Part print with two shaded views. Sizes in mm from the minimum x, y, z corner. A direction names the side the tool comes from. Round coordinates to 2 decimals unless told otherwise and drop trailing zeros. Loops run counter-clockwise (first coordinate to the right, second up) from the corner with the lowest first, then second, coordinate; pieces in that order, holes last. Notation, with made-up numbers: M -40,73.25 L -28,73.25 A29 ccw -28,108.25 Z; hole C 73,49 d11. An arc over 180 degrees is marked long. Use a Markdown table: item, result. Add a question column.
Item 1: Saw through at C-C on z = 4.25. Write the cut outline in (x, y), then the cut area to 3 significant figures.
Item 2: Tool access for the marked faces 1 and 2: list every direction of +Z, -Z, +X, -X, +Y, -Y with a clear straight run to the whole face (end or side of a thin tool).
Item 3: Pin check, flat tip, straight feed: P1, Ø3, axis at x = 4.5, z = 5, coming from the +Y side. Stop position of the tip, or through.
Item 4: Saw through at A-A on y = 2.6. Write the cut outline in (x, z).
Item 5: Wall check: L1, parallel to Y at x = 2.5, z = 6.5; L2, parallel to Z at x = 4.95, y = 1.6; L3, parallel to Y at x = 4.9, z = 2.75. Give the ranges that are in metal, low to high. Write a range as from..to.
Item 6: Saw through at D-D on z = 5.5. Write the cut outline in (x, y).
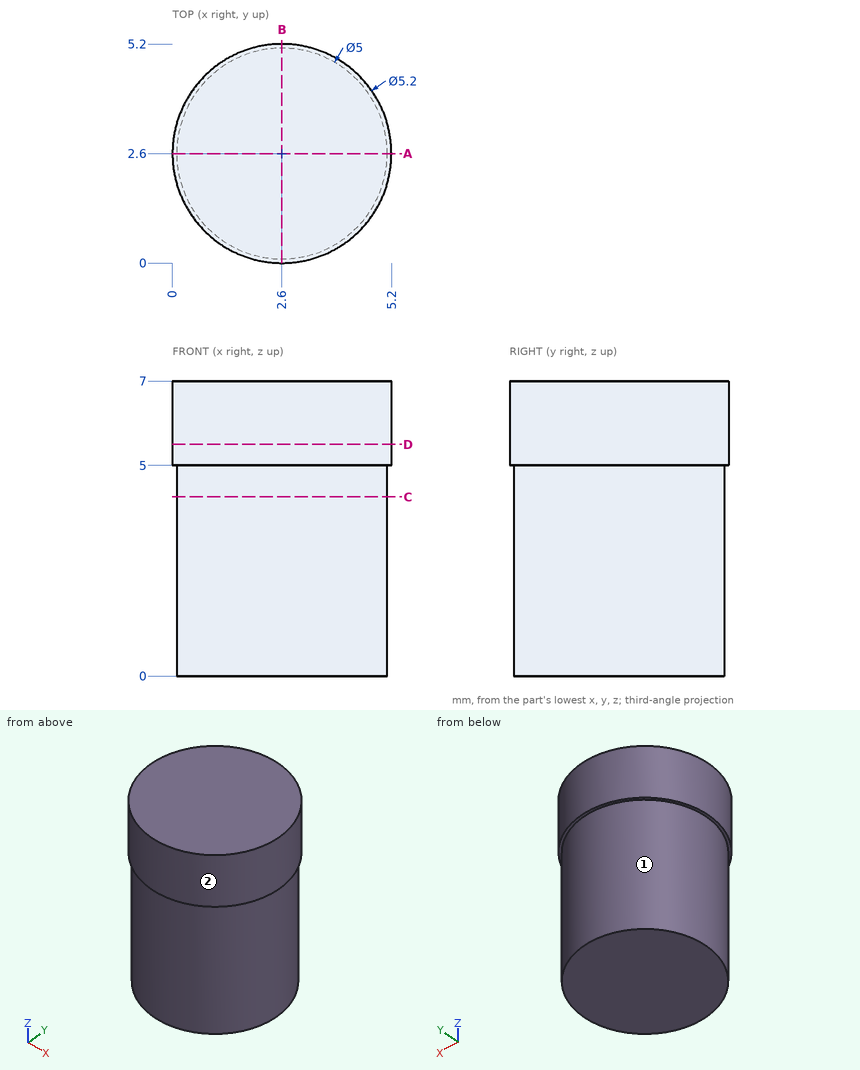
Entries:
| question | item | result |
|---|---|---|
| 1 | outline | C 2.6,2.6 d5 |
| 1 | area | 19.6 mm2 |
| 2 | face 1 | -Z |
| 2 | face 2 | +Z, -Z |
| 3 | P1 | y = 5.17 |
| 4 | outline | M 0,5 L 0.1,5 L 0.1,0 L 5.1,0 L 5.1,5 L 5.2,5 L 5.2,7 L 0,7 Z |
| 5 | L1 | 0..5.2 |
| 5 | L2 | 5..7 |
| 5 | L3 | 1.62..3.58 |
| 6 | outline | C 2.6,2.6 d5.2 |
